Could you check a few things on this drawing? It's one solid part, dimensions in mm from its lowest x, y, z. Give positions to 0.01 mm unless a question says otherwise; leave off trailing zeros. Loops run counter-clockwise (first coordinate to the right, second up) from the corner with the lowest first, then second, coordinate; pieces in that order, holes last. Notation, with made-up numbers: (60.25, 60.5) - (116.25, 60.5) arc R17 ccw to (116.25, 92.5) - close; hole circle Ø10 at (4.5, 86). An arc over 180 degrees is marked (long way). Answer as a JSON object with one key per item and string values.
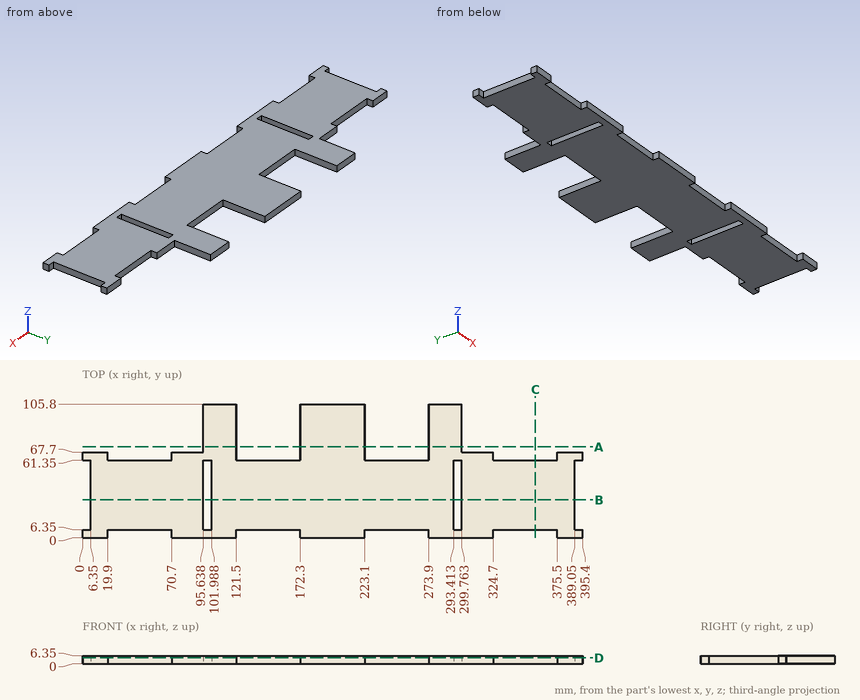
1) Imagine slicing it at C-C on x = 358. Write out the boundary of the cut face in (y, z).
Check sheet entries:
{"outline": "(6.35, 0) - (61.35, 0) - (61.35, 6.35) - (6.35, 6.35) - close"}
2) Imagine slicing it at A-A on y = 72. Write out the boundary of the cut face in (x, z).
Check sheet entries:
{"outline": "(95.64, 0) - (121.5, 0) - (121.5, 6.35) - (95.64, 6.35) - close; (172.3, 0) - (223.1, 0) - (223.1, 6.35) - (172.3, 6.35) - close; (273.9, 0) - (299.76, 0) - (299.76, 6.35) - (273.9, 6.35) - close"}
3) Imagine slicing it at B-B on y = 30. Write out the boundary of the cut face in (x, z).
Check sheet entries:
{"outline": "(6.35, 0) - (95.64, 0) - (95.64, 6.35) - (6.35, 6.35) - close; (101.99, 0) - (293.41, 0) - (293.41, 6.35) - (101.99, 6.35) - close; (299.76, 0) - (389.05, 0) - (389.05, 6.35) - (299.76, 6.35) - close"}
4) I'm going to push flat-ended pins straight in: P1, Ø3, axis at x = 385, z = 2.5, coming from the +Y side; P2, Ø1.9, axis at y = 73, z = 2, coming from the -X side; P3, Ø2, axis at x = 68.5, z = 1.5, coming from the +Y side. Where does each tip first touch, or does it pass through?
Check sheet entries:
{"P1": "y = 67.7", "P2": "x = 95.64", "P3": "y = 61.35"}
5) I need wall thicknesses on L1, parallel to X at y = 54, z = 1; L2, parallel to X at y = 75, z = 3.75; L3, parallel to Y at x = 363.5, z = 1. Which ranges of each line are inside material? Lowest first, please.
Check sheet entries:
{"L1": "6.35 to 95.64, 101.99 to 293.41, 299.76 to 389.05", "L2": "95.64 to 121.5, 172.3 to 223.1, 273.9 to 299.76", "L3": "6.35 to 61.35"}
6) Imagine slicing it at D-D on z = 4.75. Give the number of separate pieces and of enclosed holes in the cut face, and give its area (3 significant figures).
Check sheet entries:
{"separate pieces": "1", "enclosed holes": "2", "area": "26,700 mm2"}
